CAD build for the part. Positions are in the model's coordinates, mm. A direction names the side the tool comes from. Round coordinates to 2 decimals unless told otherwise and drop trailing zeros. Write each loop counter-clockwise with the first axis right and the second up, starting at its lowest first coordinate (ties: lowest second). Pieces come first, ordered by that corner, then holes. Notation, with made-up numbers: (-8, 14.5) - (2, 14.5) arc R33 cw to (2, 43.5) - close; hole circle Ø1 at (44, 44.25). An arc over 180 degrees is marked (long way). Use one line per item in the form item = value. Start each with the question number.
Item 1: Band-saw the part on D-D, the plane z = 433. List the corners of the cut face in (x, y).
Item 2: Drill centre lines: L1, parallel to X at y = 341.5, z = 320; L2, parallel to X at y = 1108, z = 146.5; L3, parallel to Z at x = 551, y = 942. Where is each one in solid material? Low to high.
Item 3: Tool access for faces 4 (the flat face through (771, 1562, 495.3)), 5 (the flat face through (75, 106, 285.75)), 6 (the flat face through (145, 1316, 260.35)): list every direction of +Z, -Z, +X, -X, +Y, -Y with a clear straight run to the whole face (end or side of a thin tool).
Item 4: Pull direction Y, two halves, no side cores. Call faces 1 (the flat face through (145, 926, 285.75)), 2 (the flat face through (714, 0, 26)), 3 (the flat face through (1473.2, 441, 167)): +Y half, -Y half, draft (parallel to the pull), parting line (faces both ways), or undercut.
Item 5: Pin check, flat tips, straight feed: pin 1 (1 mm diameter, centred on y = 633, z = 130.5, fed in from -X); pin 2 (12 mm diameter, centred on x = 554, z = 222, fed in from -Y); pin 3 (12.5 mm diameter, centred on x = 67.5, y = 367.5, fed in from +Z); pin 4 (6 mm diameter, centred on x = 461.5, y = 1034, fed in from +Z). Stop position of each tip, or through.
Item 6: Band-saw the part on B-B, the plane y = 1360. List the corners of the cut face in (x, z), and give its area (3 significant figures).
Item 7: Band-saw the part on C-C, the plane x = 1153. List the corners of the cut face in (y, z), and give its area (3 significant figures).
from build123d import *

# Parameters (mm, degrees)
F0_W     = 1549.4
F0_H     = 1587.5
F1_DEPTH = 495.3
F2_W     = 1447.8
F2_H     = 1536.7
F3_DEPTH = 209.55
F5_DEPTH = 241.3
F6_SIZE  = 165.09999
F7_SIZE  = 165.09999
F8_W     = 192.0828819275
F8_H     = 165.1
F8_W_2   = 25.4
F8_W_3   = 25.217294693
F8_W_4   = 190.5
F9_DEPTH = 25.4


# Not quite as in the source:
# - a fillet or chamfer is up to 0.001 mm smaller than in the source, because OpenCascade refuses the exact size


with BuildPart() as f1:
    # F0 (on Top) → F1 (new body)
    with BuildSketch(Plane.XY):
        with Locations((774.7, 793.75)):
            Rectangle(F0_W, F0_H)
    extrude(amount=F1_DEPTH)

    # F2 (on face) → F3 (cut)
    with BuildSketch(Plane.XY.offset(495.3)):
        with Locations((774.7, 768.35)):
            Rectangle(F2_W, F2_H)
    extrude(amount=-F3_DEPTH, mode=Mode.SUBTRACT)

    # F4 (on face) → F5 (cut)
    with BuildSketch(Plane.XY.offset(285.75)):
        Polygon((114.3, 101.6), (114.3, 0), (1435.1, 0), (1435.1, 101.6), (1473.2, 215.9), (1473.2, 673.1), (1308.1, 673.1), (1308.1, 1536.7), (241.3, 1536.7), (241.3, 673.1), (76.2, 673.1), (76.2, 215.9), align=None)
    extrude(amount=-F5_DEPTH, mode=Mode.SUBTRACT)

    # F6 (size 165.1 in the source; OpenCascade refuses exactly that, so slightly less here)
    f6_edges = [f1.edges().sort_by_distance(p)[0] for p in [
        (241.3, 673.1, 165.1),
    ]]
    chamfer(f6_edges, length=F6_SIZE)

    # F7 (size 165.1 in the source; OpenCascade refuses exactly that, so slightly less here)
    f7_edges = [f1.edges().sort_by_distance(p)[0] for p in [
        (1308.1, 673.1, 165.1),
    ]]
    chamfer(f7_edges, length=F7_SIZE)

    # F8 (on face) → F9 (cut)
    with BuildSketch(Plane.XY.offset(285.75)):
        with Locations((1403.493642807, 1314.45)):
            Rectangle(F8_W, F8_H)
        with Locations((63.5, 349.25)):
            Rectangle(F8_W_2, F8_H)
        with Locations((1485.9412908554, 349.25)):
            Rectangle(F8_W_3, F8_H)
        with Locations((146.05, 1314.45)):
            Rectangle(F8_W_4, F8_H)
    extrude(amount=-F9_DEPTH, mode=Mode.SUBTRACT)


solid = f1.part
Determined:
q1.outline = (0, 0) - (50.8, 0) - (50.8, 1536.7) - (1498.6, 1536.7) - (1498.6, 0) - (1549.4, 0) - (1549.4, 1587.5) - (0, 1587.5) - close
q2.L1 = 0 to 50.8, 1498.6 to 1549.4
q2.L2 = 0 to 241.3, 1308.1 to 1549.4
q2.L3 = 0 to 44.45
q3.face_4 = +Z, +X, -X, +Y, -Y
q3.face_5 = +Z, -Y
q3.face_6 = +Z
q4.face_1 = draft
q4.face_2 = -Y half
q4.face_3 = undercut
q5.pin_1 = 0
q5.pin_2 = 1536.7
q5.pin_3 = 260.35
q5.pin_4 = 44.45
q6.outline = (0, 0) - (1549.4, 0) - (1549.4, 495.3) - (1498.6, 495.3) - (1498.6, 285.75) - (1499.54, 285.75) - (1499.54, 260.35) - (1308.1, 260.35) - (1308.1, 44.45) - (241.3, 44.45) - (241.3, 260.35) - (50.8, 260.35) - (50.8, 495.3) - (0, 495.3) - close
q6.area = 197,000 mm²
q7.outline = (0, 0) - (1587.5, 0) - (1587.5, 495.3) - (1536.7, 495.3) - (1536.7, 44.45) - (0, 44.45) - close
q7.area = 93,500 mm²
